Design review of the part built by this model. Coordinates are the model's own, in mm. A direction names the side the tool comes from. Round coordinates to 2 decimals unless told otherwise and drop trailing zeros. Loops run counter-clockwise (first coordinate to the right, second up) from the corner with the lowest first, then second, coordinate; pieces in that order, holes last. Notation, with made-up numbers: (22.5, -5.5) -> (72.5, -5.5) arc R27 cw to (72.5, 16.5) -> close; hole circle Ø5 at (40, 41.25). An arc over 180 degrees is marked (long way). Use a Markdown table: item, result. Add a question column.
from build123d import *

# Parameters (mm, degrees)
SKETCH_1_R          = 9
EXTRUDE_1_DEPTH     = 25
SKETCH_2_R          = 4
CUT_EXTRUDE_1_DEPTH = 20
SKETCH_6_R          = 6
EXTRUDE_4_DEPTH     = 19.5
SKETCH_3_W          = 8
SKETCH_3_H          = 8
EXTRUDE_2_DEPTH     = 8
SKETCH_4_R          = 4
EXTRUDE_3_DEPTH     = 20
SKETCH_5_R          = 1.5
CUT_EXTRUDE_2_DEPTH = 74.608763065
CHAMFER_1_SIZE      = 1
SKETCH_7_W          = 0.5
SKETCH_7_H          = 0.8


with BuildPart() as part:
    # 草图1 → 凸台-拉伸1 (new body)
    with BuildSketch(Plane(origin=(0, 0, 0), x_dir=(1, 0, 0), z_dir=(0, 1, 0))):
        with Locations(Location((0, 0, 0), (0, 0, 270))):
            Circle(SKETCH_1_R)
    extrude(amount=EXTRUDE_1_DEPTH)

    # 草图2 → 切除-拉伸1 (cut)
    with BuildSketch(Plane.XZ):
        with Locations(Location((0, 0, 0), (0, 0, 270))):
            Circle(SKETCH_2_R)
    extrude(amount=-CUT_EXTRUDE_1_DEPTH, mode=Mode.SUBTRACT)

    # 草图6 → 凸台-拉伸4 (add)
    with BuildSketch(Plane(origin=(0, 25, 0), x_dir=(1, 0, 0), z_dir=(0, 1, 0))):
        with Locations(Location((0, 0, 0), (0, 0, 270))):
            Circle(SKETCH_6_R)
    extrude(amount=EXTRUDE_4_DEPTH)

    # 草图3 → 凸台-拉伸2 (add)
    with BuildSketch(Plane(origin=(0, 44.5, 0), x_dir=(1, 0, 0), z_dir=(0, 1, 0))):
        Rectangle(SKETCH_3_W, SKETCH_3_H)
    extrude(amount=EXTRUDE_2_DEPTH)

    # 草图4 → 凸台-拉伸3 (add)
    with BuildSketch(Plane(origin=(0, 52.5, 0), x_dir=(1, 0, 0), z_dir=(0, 1, 0))):
        with Locations(Location((0, 0, 0), (0, 0, 90))):
            Circle(SKETCH_4_R)
    extrude(amount=EXTRUDE_3_DEPTH)

    # 草图5 → 切除-拉伸2 (cut, through all)
    with BuildSketch(Plane(origin=(0, 0, 0), x_dir=(0, 0, -1), z_dir=(1, 0, 0))):
        with Locations((0, 10)):
            Circle(SKETCH_5_R)
    extrude(amount=-CUT_EXTRUDE_2_DEPTH, mode=Mode.SUBTRACT)

    # 倒角1
    chamfer_1_edges = [part.edges().sort_by_distance(p)[0] for p in [
        (0, 72.5, 4),
    ]]
    chamfer(chamfer_1_edges, length=CHAMFER_1_SIZE)

    # 草图7 → 切除-旋转1 (revolve, cut)
    with BuildSketch(Plane(origin=(0, 0, 0), x_dir=(0, 0, -1), z_dir=(1, 0, 0)), mode=Mode.PRIVATE) as cut_revolve_1_sk:
        with Locations((3.75, 62.9)):
            Rectangle(SKETCH_7_W, SKETCH_7_H)
        with Locations((3.75, 52.9)):
            Rectangle(SKETCH_7_W, SKETCH_7_H)
    revolve(cut_revolve_1_sk.sketch.rotate(Axis((0, 72.5, 0), (0, -1, 0)), 180), axis=Axis((0, 72.5, 0), (0, -1, 0)), mode=Mode.SUBTRACT)


solid = part.part
1. Insertion check: P1, Ø8, axis at x = 4.5, y = 43, coming from the -Z side; P2, Ø2.5, axis at x = 1.5, z = 1, coming from the -Y side; P3, Ø6.5, axis at x = -2, y = 47, coming from the +Z side; P4, Ø6, axis at x = 3.5, z = -4.5, coming from the +Y side. Each pin has a flat end and moves straight along its axis. Give the tip position at first contact, or say it passes through.
2. Consider section D-D on x = -7. State the section outline as (y, z) points.
3. Consider section C-C on y = 36. State the section outline as (x, z) points.
4. For faces 4 (the face through (0, 48, -4)), 5 (the face through (-6, 25, 2)), 6 (the face through (1.341, 52.906, 3.233)), list the 3-axis set-ups (+Z, -Z, +X, -X, +Y, -Y) from which the entire face can be reached by the end or side of a thin tool; tool diameter is ignored.
5. To check wall thickness, follow probe 1 along X at (y, z) = (8, -0.25); probe 2 along Y at (x, z) = (-7.2, 0); probe 3 along Y at (x, z) = (-2, 0.25). State the ranges of each line that lie inside material, in increasing order. Write a range as from..to.
6. Consider section B-B on y = 5. State the section outline as (x, z) points.
7. Mouldability with a two-part tool opening along Y and no side actions: class faces 1 (the face through (3.905, 57.836, 0.867)), 2 (the face through (-6.318, 9.425, -1.386)), 3 (the face through (0, 20, 0)) as +Y half, -Y half, draft (parallel to the pull), parting line (faces both ways), or undercut.
Verdict:
| question | item | result |
|---|---|---|
| 1 | P1 | stops at z = -5.98 |
| 1 | P2 | stops at y = 20 |
| 1 | P3 | stops at z = 6 |
| 1 | P4 | stops at y = 72.5 |
| 2 | outline | (0, -5.66) -> (25, -5.66) -> (25, 5.66) -> (0, 5.66) -> close; hole circle Ø3 at (10, 0) |
| 3 | outline | circle Ø12 at (0, 0) |
| 4 | face 4 | -Z, +X, -X, +Y |
| 4 | face 5 | +Y |
| 4 | face 6 | none |
| 5 | probe 1 | x = -9..-3.99, 3.99..9 |
| 5 | probe 2 | y = 0..8.5, 11.5..25 |
| 5 | probe 3 | y = 20..72.5 |
| 6 | outline | circle Ø18 at (0, 0); hole circle Ø8 at (0, 0) |
| 7 | face 1 | draft |
| 7 | face 2 | undercut |
| 7 | face 3 | -Y half |
